Input: part model. Units: mm. Frame: model coordinates. A direction names the side the tool comes from. Give positions to 0.01 mm unless a question says otherwise; leave off trailing zeros. Loops run counter-clockwise (first coordinate to the right, second up) from the corner with the lowest first, then second, coordinate; pieces in that order, holes last.
from build123d import *

# Parameters (mm, degrees)
SKETCH2_R               = 9
BOSS_EXTRUDE1_DEPTH     = 20
CUT_EXTRUDE1_DEPTH      = 20
SKETCH4_R               = 50
SKETCH4_R_2             = 4.5
BOSS_EXTRUDE3_DEPTH     = 5
CUT_EXTRUDE2_DEPTH      = 9
CUT_EXTRUDE2_DEPTH_BACK = 9
SKETCH11_R              = 1.55
CUT_EXTRUDE9_DEPTH      = 9
CUT_EXTRUDE9_DEPTH_BACK = 9
SKETCH15_R              = 1.55
SKETCH28_R              = 5
SKETCH28_R_2            = 4
SKETCH28_R_3            = 1.55
BOSS_EXTRUDE10_DEPTH    = 3
SKETCH25_R              = 17
SKETCH25_R_2            = 8
BOSS_EXTRUDE8_DEPTH     = 5
SKETCH26_R              = 1.55
CUT_EXTRUDE14_DEPTH     = 8
SKETCH27_R              = 3
CUT_EXTRUDE15_DEPTH     = 3
SKETCH16_R              = 1.55
CUT_EXTRUDE17_DEPTH     = 5
SKETCH29_R              = 3
CUT_EXTRUDE18_DEPTH     = 3
SKETCH30_R              = 17
SKETCH30_R_2            = 9.5
BOSS_EXTRUDE11_DEPTH    = 6
CUT_EXTRUDE23_START     = 9
SKETCH31_R              = 3
CUT_EXTRUDE23_DEPTH     = 2.5
CUT_EXTRUDE24_START     = -6.5
SKETCH31_3_R            = 3
CUT_EXTRUDE24_DEPTH     = 2.5
CUT_EXTRUDE25_START     = 9
SKETCH33_R              = 3
CUT_EXTRUDE25_DEPTH     = 2.5
CUT_EXTRUDE26_START     = -6.5
SKETCH33_2_R            = 3
CUT_EXTRUDE26_DEPTH     = 2.5


with BuildPart() as part:
    # Sketch2 → Boss-Extrude1 (new body)
    with BuildSketch(Plane(origin=(0, 0, 0), x_dir=(1, 0, 0), z_dir=(0, 1, 0))):
        with Locations(Location((0, 0, 0), (0, 0, 270))):
            Circle(SKETCH2_R)
    extrude(amount=BOSS_EXTRUDE1_DEPTH)

    # Sketch3 → Cut-Extrude1 (cut)
    with BuildSketch(Plane(origin=(0, 20, 0), x_dir=(1, 0, 0), z_dir=(0, 1, 0))):
        Polygon((0, 4), (-3.464101615, 2), (-3.464101615, -2), (0, -4), (3.464101615, -2), (3.464101615, 2), align=None)
    extrude(amount=-CUT_EXTRUDE1_DEPTH, mode=Mode.SUBTRACT)

    # Sketch4 → Boss-Extrude3 (add)
    with BuildSketch(Plane(origin=(0, 20, 0), x_dir=(1, 0, 0), z_dir=(0, 1, 0))):
        with Locations(Location((0, 0, 0), (0, 0, 270))):
            Circle(SKETCH4_R)
        Circle(SKETCH4_R_2, mode=Mode.SUBTRACT)
    extrude(amount=-BOSS_EXTRUDE3_DEPTH)

    # Sketch11 → Cut-Extrude2 (cut, two sides: drawn at the far end of the back side and taken through both)
    with BuildSketch(Plane(origin=(0, 0, 0), x_dir=(0.8660254037844384, 0, -0.5000000000000006), z_dir=(0.5000000000000006, 0, 0.8660254037844384)).offset(-CUT_EXTRUDE2_DEPTH_BACK)):
        with Locations(Location((0, 5, 0), (0, 0, 180))):
            Circle(SKETCH11_R)
    extrude(amount=CUT_EXTRUDE2_DEPTH + CUT_EXTRUDE2_DEPTH_BACK, mode=Mode.SUBTRACT)

    # Sketch15 → Cut-Extrude9 (cut, two sides: drawn at the far end of the back side and taken through both)
    with BuildSketch(Plane(origin=(0, 0, 0), x_dir=(0, 0, -1), z_dir=(1, 0, 0)).offset(-CUT_EXTRUDE9_DEPTH_BACK)):
        with Locations(Location((0, 9, 0), (0, 0, 270))):
            Circle(SKETCH15_R)
    extrude(amount=CUT_EXTRUDE9_DEPTH + CUT_EXTRUDE9_DEPTH_BACK, mode=Mode.SUBTRACT)

    # Sketch28 → Boss-Extrude10 (add)
    with BuildSketch(Plane.ZY.offset(32)):
        with BuildLine():
            Line((25, 15), (-25, 15))
            Line((-25, 15), (-17, -135))
            ThreePointArc((-17, -135), (0, -152), (17, -135))
            Line((17, -135), (25, 15))
        make_face()
        with Locations((0, -135)):
            Circle(SKETCH28_R, mode=Mode.SUBTRACT)
        with Locations((0, -75)):
            Circle(SKETCH28_R_2, mode=Mode.SUBTRACT)
        with Locations((7.186666667, -46.5)):
            Circle(SKETCH28_R_3, mode=Mode.SUBTRACT)
        with Locations((-7.186666667, -46.5)):
            Circle(SKETCH28_R_3, mode=Mode.SUBTRACT)
    extrude(amount=BOSS_EXTRUDE10_DEPTH)

    # Sketch25 → Boss-Extrude8 (add)
    with BuildSketch(Plane.ZY.offset(35)):
        with Locations((0, -135)):
            Circle(SKETCH25_R)
        with Locations((0, -135)):
            Circle(SKETCH25_R_2, mode=Mode.SUBTRACT)
    extrude(amount=BOSS_EXTRUDE8_DEPTH)

    # Sketch26 → Cut-Extrude14 (cut)
    with BuildSketch(Plane.ZY.offset(40)):
        with Locations((-12.5, -135)):
            Circle(SKETCH26_R)
        with Locations((0, -122.5)):
            Circle(SKETCH26_R)
        with Locations((12.5, -135)):
            Circle(SKETCH26_R)
        with Locations((0, -147.5)):
            Circle(SKETCH26_R)
    extrude(amount=-CUT_EXTRUDE14_DEPTH, mode=Mode.SUBTRACT)

    # Sketch27 → Cut-Extrude15 (cut)
    with BuildSketch(Plane(origin=(-32, 0, 0), x_dir=(0, 0, -1), z_dir=(1, 0, 0))):
        with Locations((-12.5, -135)):
            Circle(SKETCH27_R)
        with Locations((0, -122.5)):
            Circle(SKETCH27_R)
        with Locations((12.5, -135)):
            Circle(SKETCH27_R)
        with Locations((0, -147.5)):
            Circle(SKETCH27_R)
    extrude(amount=-CUT_EXTRUDE15_DEPTH, mode=Mode.SUBTRACT)

    # Sketch16 → Cut-Extrude17 (cut)
    with BuildSketch(Plane.XZ.offset(-15)):
        with Locations(Location((29.154127235, 12.5, 0), (0, 0, 270))):
            Circle(SKETCH16_R)
        with Locations(Location((29.154127235, 0, 0), (0, 0, 270))):
            Circle(SKETCH16_R)
        with Locations(Location((29.154127235, -12.5, 0), (0, 0, 270))):
            Circle(SKETCH16_R)
        with Locations(Location((38, -12.5, 0), (0, 0, 270))):
            Circle(SKETCH16_R)
        with Locations(Location((38, 0, 0), (0, 0, 270))):
            Circle(SKETCH16_R)
        with Locations(Location((38, 12.5, 0), (0, 0, 270))):
            Circle(SKETCH16_R)
    extrude(amount=-CUT_EXTRUDE17_DEPTH, mode=Mode.SUBTRACT)

    # Sketch29 → Cut-Extrude18 (cut)
    with BuildSketch(Plane(origin=(0, 20, 0), x_dir=(1, 0, 0), z_dir=(0, 1, 0))):
        with Locations(Location((29.154127235, 12.5, 0), (0, 0, 270))):
            Circle(SKETCH29_R)
        with Locations(Location((38.154127235, 12.5, 0), (0, 0, 270))):
            Circle(SKETCH29_R)
        with Locations(Location((38.154127235, 0, 0), (0, 0, 270))):
            Circle(SKETCH29_R)
        with Locations(Location((38.154127235, -12.5, 0), (0, 0, 270))):
            Circle(SKETCH29_R)
        with Locations(Location((29.154127235, 0, 0), (0, 0, 270))):
            Circle(SKETCH29_R)
        with Locations(Location((29.154127235, -12.5, 0), (0, 0, 270))):
            Circle(SKETCH29_R)
    extrude(amount=-CUT_EXTRUDE18_DEPTH, mode=Mode.SUBTRACT)

    # Sketch30 → Boss-Extrude11 (add)
    with BuildSketch(Plane.ZY.offset(35)):
        with Locations(Location((0, -75, 0), (0, 0, 180))):
            Circle(SKETCH30_R)
        with Locations((0, -75)):
            Circle(SKETCH30_R_2, mode=Mode.SUBTRACT)
    extrude(amount=BOSS_EXTRUDE11_DEPTH)

    # Sketch31 → Cut-Extrude23 (cut)
    with BuildSketch(Plane(origin=(0, 0, 0), x_dir=(0.8660254037844384, 0, -0.5000000000000006), z_dir=(0.5000000000000006, 0, 0.8660254037844384)).offset(CUT_EXTRUDE23_START)):
        with Locations((0, 5)):
            Circle(SKETCH31_R)
    extrude(amount=-CUT_EXTRUDE23_DEPTH, mode=Mode.SUBTRACT)

    # Sketch31_3 → Cut-Extrude24 (cut)
    with BuildSketch(Plane(origin=(0, 0, 0), x_dir=(0.8660254037844384, 0, -0.5000000000000006), z_dir=(0.5000000000000006, 0, 0.8660254037844384)).offset(CUT_EXTRUDE24_START)):
        with Locations((0, 5)):
            Circle(SKETCH31_3_R)
    extrude(amount=-CUT_EXTRUDE24_DEPTH, mode=Mode.SUBTRACT)

    # Sketch33 → Cut-Extrude25 (cut)
    with BuildSketch(Plane(origin=(0, 0, 0), x_dir=(0, 0, -1), z_dir=(1, 0, 0)).offset(CUT_EXTRUDE25_START)):
        with Locations(Location((0, 9, 0), (0, 0, 90))):
            Circle(SKETCH33_R)
    extrude(amount=-CUT_EXTRUDE25_DEPTH, mode=Mode.SUBTRACT)

    # Sketch33_2 → Cut-Extrude26 (cut)
    with BuildSketch(Plane(origin=(0, 0, 0), x_dir=(0, 0, -1), z_dir=(1, 0, 0)).offset(CUT_EXTRUDE26_START)):
        with Locations(Location((0, 9, 0), (0, 0, 90))):
            Circle(SKETCH33_2_R)
    extrude(amount=-CUT_EXTRUDE26_DEPTH, mode=Mode.SUBTRACT)


solid = part.part
(1) Reachability of faces 1 (the flat face through (-2.132, 3.709, -6.275)), 2 (the cylindrical face through (-33.48, -132.47, -14.11)), 3 (the cylindrical face through (-37.47, -142.81, -1.73)), 4 (the flat face through (-1.708, 10.14, -3.014)) from +Z, -Z, +X, -X, +Y, -Y: full face, straight path, thin tool, end or side. Return the list, or none.
Values follow:
face 1: none
face 2: +X
face 3: -X
face 4: +Y, -Y
(2) Pin query (flat end, axial travel): pin 1 Ø3 at (x, z) = (38, 12.5) entering from -Y; pin 2 Ø2.5 at (y, z) = (9, 0) entering from -X; pin 3 Ø10 at (x, z) = (-22, 34.5) entering from -Y; pin 4 Ø3 at (y, z) = (-121, 0.5) entering from +X. Return the tip coordinate at first contact, or that it passes through.
Values follow:
pin 1: passes through
pin 2: stops at x = -35
pin 3: stops at y = 15
pin 4: stops at x = -32
(3) Cut plane C-C (z = 22). Return the cut outline in (x, y).
Values follow:
outline: (-44.9, 15) - (-35, 15) - (-35, -41.25) - (-32, -41.25) - (-32, 15) - (44.9, 15) - (44.9, 20) - (-44.9, 20) - close
(4) Cut plane B-B (x = 19.5). Return the cut outline in (y, z).
Values follow:
outline: (15, -46.04) - (20, -46.04) - (20, 46.04) - (15, 46.04) - close
(5) Ray query, probe 1 along Y at (x, z) = (-32.55, 0); probe 2 along Z at (x, y) = (4.2, 9); probe 3 along X at (y, z) = (19, -12). Return the intervals inside material, ascending.
Values follow:
probe 1: y = -152 to -150.5, -144.5 to -140, -130 to -125.5, -119.5 to -79, -71 to 20
probe 2: z = -7.96 to -1.55, 1.55 to 7.96
probe 3: x = -48.54 to 26.2, 32.11 to 35.2, 41.11 to 48.54
(6) Mould query, pull axis Z, two halves, no side actions, for faces 5 (the flat face through (-4, 0, 0)), 6 (the flat face through (39, 17, -11)), 7 (the cylindrical face through (-36.833, -151.596, -3.685)). Classes: +Z half, -Z half, draft (parallel to the pull), parting line (faces both ways), or undercut.
Values follow:
face 5: draft
face 6: undercut
face 7: parting line
(7) Cut plane A-A (z = 40). Return the cut outline in (x, y).
Values follow:
outline: (-30, 15) - (30, 15) - (30, 20) - (-30, 20) - close
